Work out the finished part from the listing and answer in its coordinate system (mm). Give positions to 0.01 mm unless a question says otherwise; leave off trailing zeros. Order: outer loops, then holes, each group sorted by start corner. A loop starts at its lowest first (then second) coordinate and runs counter-clockwise, first axis right, second up. Notation, with made-up numbers: (12, 69) - (16, 69) arc R20 ccw to (16, 99) - close; hole circle Ø4 at (18, 42.5). An arc over 180 degrees is marked (long way). Return JSON: item names as keys, results as strings. Group by question number.
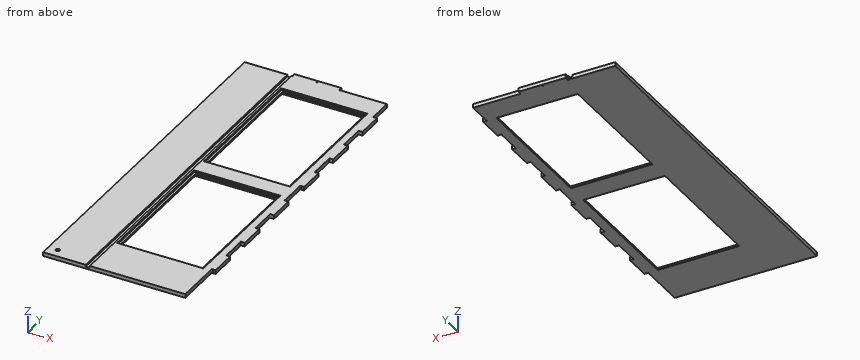
from build123d import *

# Parameters (mm, degrees)
ESQUISSE1_R             = 1
ESQUISSE1_W             = 172
ESQUISSE1_H             = 281.553390594
ESQUISSE1_H_2           = 280.534461641
BOSS_EXTRU_1_DEPTH      = 8
ENL_V_MAT_EXTRU_1_DEPTH = 4
ESQUISSE3_W             = 8.5
ESQUISSE3_H             = 760.715269233
ENL_V_MAT_EXTRU_2_DEPTH = 4
ESQUISSE4_R             = 4
ENL_V_MAT_EXTRU_3_DEPTH = 6


with BuildPart() as part:
    # Esquisse1 → Boss.-Extru.1 (new body)
    with BuildSketch(Plane.XY):
        with BuildLine():
            Line((-54.650090097, -45.819197646), (-54.650090097, 358.028972494))
            Line((-54.650090097, 358.028972494), (-54.650090097, 714.896071587))
            Line((-54.650090097, 714.896071587), (43.228589559, 714.896071587))
            ThreePointArc((43.228589559, 714.896071587), (45.349909903, 714.896071587), (45.349909903, 717.01739193))
            Line((45.349909903, 717.01739193), (45.349909903, 722.896071587))
            Line((45.349909903, 722.896071587), (145.349909903, 722.896071587))
            Line((145.349909903, 722.896071587), (145.349909903, 717.01739193))
            ThreePointArc((145.349909903, 717.01739193), (145.349909903, 714.896071587), (147.471230246, 714.896071587))
            Line((147.471230246, 714.896071587), (245.349909903, 714.896071587))
            Line((245.349909903, 714.896071587), (245.349909903, 665.01739193))
            ThreePointArc((245.349909903, 665.01739193), (245.349909903, 662.896071587), (247.471230246, 662.896071587))
            Line((247.471230246, 662.896071587), (253.349909903, 662.896071587))
            Line((253.349909903, 662.896071587), (253.349909903, 607.896071587))
            Line((253.349909903, 607.896071587), (247.471230246, 607.896071587))
            ThreePointArc((247.471230246, 607.896071587), (245.349909903, 607.896071587), (245.349909903, 605.774751243))
            Line((245.349909903, 605.774751243), (245.349909903, 555.01739193))
            ThreePointArc((245.349909903, 555.01739193), (245.349909903, 552.896071587), (247.471230246, 552.896071587))
            Line((247.471230246, 552.896071587), (253.349909903, 552.896071587))
            Line((253.349909903, 552.896071587), (253.349909903, 497.896071587))
            Line((253.349909903, 497.896071587), (247.471230246, 497.896071587))
            ThreePointArc((247.471230246, 497.896071587), (245.349909903, 497.896071587), (245.349909903, 495.774751243))
            Line((245.349909903, 495.774751243), (245.349909903, 445.01739193))
            ThreePointArc((245.349909903, 445.01739193), (245.349909903, 442.896071587), (247.471230246, 442.896071587))
            Line((247.471230246, 442.896071587), (253.349909903, 442.896071587))
            Line((253.349909903, 442.896071587), (253.349909903, 387.896071587))
            Line((253.349909903, 387.896071587), (247.471230246, 387.896071587))
            ThreePointArc((247.471230246, 387.896071587), (245.349909903, 387.896071587), (245.349909903, 385.774751243))
            Line((245.349909903, 385.774751243), (245.349909903, 331.302122698))
            ThreePointArc((245.349909903, 331.302122698), (245.349909903, 329.180802354), (247.471230246, 329.180802354))
            Line((247.471230246, 329.180802354), (253.349909903, 329.180802354))
            Line((253.349909903, 329.180802354), (253.349909903, 274.180802354))
            Line((253.349909903, 274.180802354), (247.471230246, 274.180802354))
            ThreePointArc((247.471230246, 274.180802354), (245.349909903, 274.180802354), (245.349909903, 272.059482011))
            Line((245.349909903, 272.059482011), (245.349909903, 221.302122698))
            ThreePointArc((245.349909903, 221.302122698), (245.349909903, 219.180802354), (247.471230246, 219.180802354))
            Line((247.471230246, 219.180802354), (253.349909903, 219.180802354))
            Line((253.349909903, 219.180802354), (253.349909903, 164.180802354))
            Line((253.349909903, 164.180802354), (247.471230246, 164.180802354))
            ThreePointArc((247.471230246, 164.180802354), (245.349909903, 164.180802354), (245.349909903, 162.059482011))
            Line((245.349909903, 162.059482011), (245.349909903, 111.302122698))
            ThreePointArc((245.349909903, 111.302122698), (245.349909903, 109.180802354), (247.471230246, 109.180802354))
            Line((247.471230246, 109.180802354), (253.349909903, 109.180802354))
            Line((253.349909903, 109.180802354), (253.349909903, 54.180802354))
            Line((253.349909903, 54.180802354), (247.471230246, 54.180802354))
            ThreePointArc((247.471230246, 54.180802354), (245.349909903, 54.180802354), (245.349909903, 52.059482011))
            Line((245.349909903, 52.059482011), (245.349909903, -45.819197646))
            Line((245.349909903, -45.819197646), (-54.650090097, -45.819197646))
        make_face()
        with Locations((95.349909903, 718.896071587)):
            Circle(ESQUISSE1_R, mode=Mode.SUBTRACT)
        with Locations((139.349909903, 522.11937629)):
            Rectangle(ESQUISSE1_W, ESQUISSE1_H, mode=Mode.SUBTRACT)
        with Locations((139.349909903, 194.448033175)):
            Rectangle(ESQUISSE1_W, ESQUISSE1_H_2, mode=Mode.SUBTRACT)
    extrude(amount=BOSS_EXTRU_1_DEPTH)

    # Esquisse2 → Enlèv. mat.-Extru.1 (cut)
    with BuildSketch(Plane.XY.offset(8)):
        with BuildLine():
            Line((50.471230246, 339.715263995), (228.228589559, 339.715263995))
            ThreePointArc((228.228589559, 339.715263995), (230.349909903, 339.715263995), (230.349909903, 337.593943652))
            Line((230.349909903, 337.593943652), (230.349909903, 51.302122698))
            ThreePointArc((230.349909903, 51.302122698), (230.349909903, 49.180802354), (228.228589559, 49.180802354))
            Line((228.228589559, 49.180802354), (50.471230246, 49.180802354))
            ThreePointArc((50.471230246, 49.180802354), (48.349909903, 49.180802354), (48.349909903, 51.302122698))
            Line((48.349909903, 51.302122698), (48.349909903, 337.593943652))
            ThreePointArc((48.349909903, 337.593943652), (48.349909903, 339.715263995), (50.471230246, 339.715263995))
        make_face()
        with BuildLine():
            Line((50.471230246, 667.896071587), (228.228589559, 667.896071587))
            ThreePointArc((228.228589559, 667.896071587), (230.349909903, 667.896071587), (230.349909903, 665.774751243))
            Line((230.349909903, 665.774751243), (230.349909903, 378.464001337))
            ThreePointArc((230.349909903, 378.464001337), (230.349909903, 376.342680993), (228.228589559, 376.342680993))
            Line((228.228589559, 376.342680993), (50.471230246, 376.342680993))
            ThreePointArc((50.471230246, 376.342680993), (48.349909903, 376.342680993), (48.349909903, 378.464001337))
            Line((48.349909903, 378.464001337), (48.349909903, 665.774751243))
            ThreePointArc((48.349909903, 665.774751243), (48.349909903, 667.896071587), (50.471230246, 667.896071587))
        make_face()
    extrude(amount=-ENL_V_MAT_EXTRU_1_DEPTH, mode=Mode.SUBTRACT)

    # Esquisse3 → Enlèv. mat.-Extru.2 (cut)
    with BuildSketch(Plane.XY.offset(8)):
        with Locations((39.599909903, 334.538436971)):
            Rectangle(ESQUISSE3_W, ESQUISSE3_H)
    extrude(amount=-ENL_V_MAT_EXTRU_2_DEPTH, mode=Mode.SUBTRACT)

    # Esquisse4 → Enlèv. mat.-Extru.3 (cut)
    with BuildSketch(Plane.XY.offset(8)):
        with Locations((-34.650090097, -25.819197646)):
            Circle(ESQUISSE4_R)
    extrude(amount=-ENL_V_MAT_EXTRU_3_DEPTH, mode=Mode.SUBTRACT)


solid = part.part
1. Consider probe 1 along X at (y, z) = (267, 4.25); probe 2 along Y at (x, z) = (186.5, 3); probe 3 along Y at (x, z) = (75, 4.75). Determine where each line is inside the solid, lowest interval first. Write a range as from..to.
2. The part is cut by section C-C (y = 32). Give the vertices of the cut face in (x, z), and give its area (3 significant figures).
3. The part is cut by section D-D (z = 6). State how many separate pieces and enclosed holes the cut face has, and give its area (3 significant figures).
4. Each of these flat-tipped pins is pushed along its axis until it touches: pin 1 (2.5 mm diameter, centred on x = 214, z = 4.5, fed in from +Y); pin 2 (1.8 mm diameter, centred on x = 249.5, z = 2.5, fed in from +Y). Where does it stop, or does it pass through?
5. The part is cut by section B-B (x = 203.5). Give the vertices of the cut face in (y, z), and give its area (3 significant figures).
6. The part is cut by section A-A (y = 264). Give the vertices of the cut face in (x, z).
Answers:
{
 "1": {"probe 1": "x = -54.65..35.35, 43.85..48.35, 230.35..245.35", "probe 2": "y = -45.82..54.18, 334.72..381.34, 662.9..714.9", "probe 3": "y = -45.82..49.18, 339.72..376.34, 667.9..722.9"},
 "2": {"outline": "(-54.65, 0) - (245.35, 0) - (245.35, 8) - (43.85, 8) - (43.85, 4) - (35.35, 4) - (35.35, 8) - (-54.65, 8) - close", "area": "2,370 mm^2"},
 "3": {"separate pieces": "2", "enclosed holes": "4", "area": "119,000 mm^2"},
 "4": {"pin 1": "stops at y = 714.9", "pin 2": "stops at y = 662.9"},
 "5": {"outline": "(-45.82, 0) - (54.18, 0) - (54.18, 4) - (49.18, 4) - (49.18, 8) - (-45.82, 8) - close; (334.72, 0) - (381.34, 0) - (381.34, 4) - (376.34, 4) - (376.34, 8) - (339.72, 8) - (339.72, 4) - (334.72, 4) - close; (662.9, 0) - (714.9, 0) - (714.9, 8) - (667.9, 8) - (667.9, 4) - (662.9, 4) - close", "area": "1,510 mm^2"},
 "6": {"outline": "(-54.65, 0) - (53.35, 0) - (53.35, 4) - (48.35, 4) - (48.35, 8) - (43.85, 8) - (43.85, 4) - (35.35, 4) - (35.35, 8) - (-54.65, 8) - close; (225.35, 0) - (245.35, 0) - (245.35, 8) - (230.35, 8) - (230.35, 4) - (225.35, 4) - close"}
}
